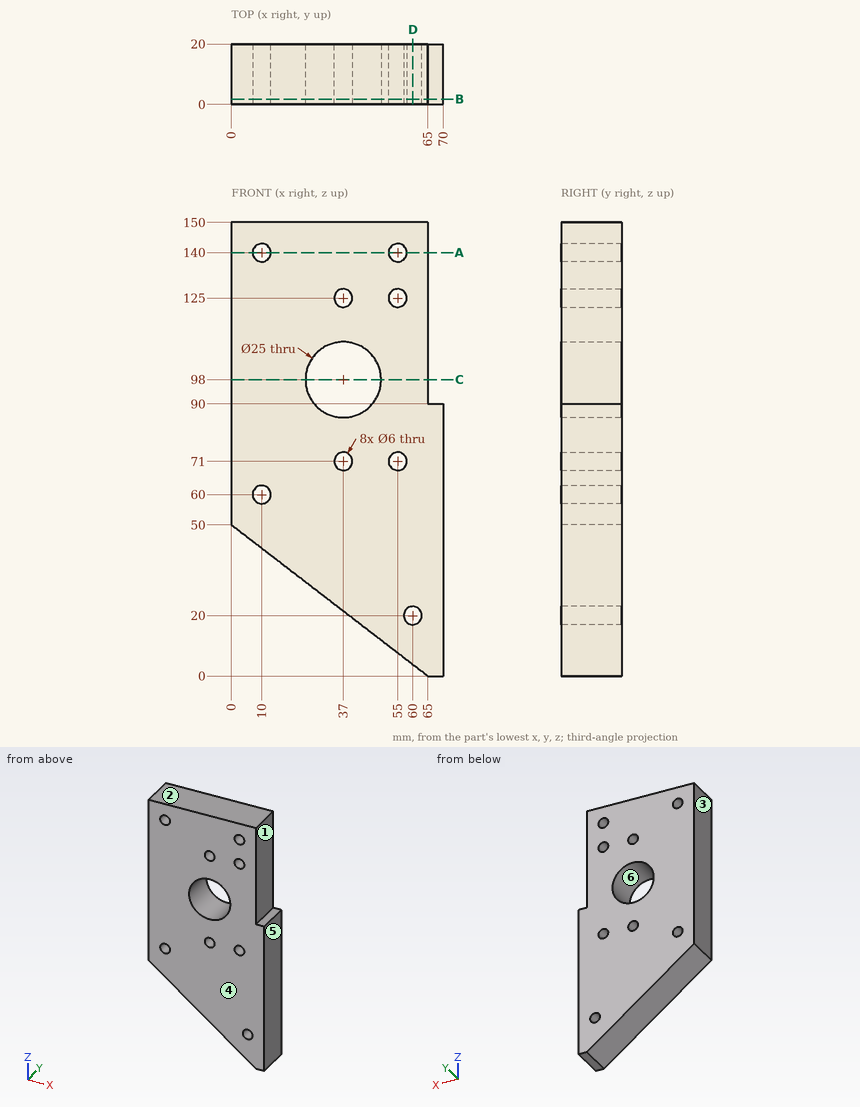
Input: dimensioned drawing with shaded views. Units: mm. Origin: part minimum x, y, z. A direction names the side the tool comes from. Give positions to 0.01 mm unless a question says otherwise; leave off trailing zeros. Write each loop counter-clockwise with the first axis right and the second up, starting at its lowest first coordinate (ties: lowest second). Pieces come first, ordered by that corner, then holes. Notation, with made-up numbers: (20, 8.25) -> (69, 8.25) arc R15 ccw to (69, 34.25) -> close; hole circle Ø5 at (48, 31.5). An arc over 180 degrees is marked (long way). Return JSON: item names as keys, results as strings. Group by question number.
1. Section C-C, the plane z = 98. Output: boundary loops of the cut face in (x, y).
2. Material intervals for line 1 (X direction, y = 4, z = 140); line 2 (Z direction, x = 37, y = 15.5); line 3 (Z direction, x = 10, y = 14.5), sorted ascending. Write a range as from..to.
3. Section A-A, the plane z = 140. Output: boundary loops of the cut face in (x, y).
4. Access query for the marked faces 1 and 2. Directions: +Z, -Z, +X, -X, +Y, -Y. A direction counts if a zero-diameter tool reaches every point of the face in a straight line with its end or side. Return the directions, or none.
5. Mould query, pull axis X, two halves, no side actions, for the marked faces 3, 4, 5 and 6. Classes: +X half, -X half, draft (parallel to the pull), parting line (faces both ways), or undercut.
6. Section D-D, the plane x = 60. Output: boundary loops of the cut face in (y, z).
7. Section B-B, the plane y = 1.75. Count the separate pieces of the cut face and the enclosed holes in it, then the cut area to 3 significant figures.
Determined:
{
 "1": {"outline": "(0, 0) -> (24.5, 0) -> (24.5, 20) -> (0, 20) -> close; (49.5, 0) -> (65, 0) -> (65, 20) -> (49.5, 20) -> close"},
 "2": {"line 1": "x = 0..7, 13..52, 58..65", "line 2": "z = 21.54..68, 74..85.5, 110.5..122, 128..150", "line 3": "z = 42.31..57, 63..137, 143..150"},
 "3": {"outline": "(0, 0) -> (7, 0) -> (7, 20) -> (0, 20) -> close; (13, 0) -> (52, 0) -> (52, 20) -> (13, 20) -> close; (58, 0) -> (65, 0) -> (65, 20) -> (58, 20) -> close"},
 "4": {"face 1": "+Z, +X, +Y, -Y", "face 2": "+Z, +X, -X, +Y, -Y"},
 "5": {"face 3": "-X half", "face 4": "draft", "face 5": "+X half", "face 6": "undercut"},
 "6": {"outline": "(0, 3.85) -> (20, 3.85) -> (20, 17) -> (0, 17) -> close; (0, 23) -> (20, 23) -> (20, 150) -> (0, 150) -> close"},
 "7": {"separate pieces": "1", "enclosed holes": "9", "area": "7,860 mm2"}
}
